Input: dimensioned drawing with shaded views. Units: mm. Origin: part minimum x, y, z. A direction names the side the tool comes from. Coordinates: 2 decimals unless noted, no trailing zeros. Loops run counter-clockwise (first coordinate to the right, second up) from the corner with the lowest first, then second, coordinate; pieces in that order, holes last.
Item 1: Line query: probe 1 along Z at (x, y) = (30.5, 32); probe 2 along Y at (x, z) = (18.5, 22); probe 3 along Z at (x, y) = (30, 19) (1 decimal). Output: solid intervals per line, ascending.
Item 2: Reachability of the marked faces 1, 2 and 3 from +Z, -Z, +X, -X, +Y, -Y: full face, straight path, thin tool, end or side. Return the list, or none.
Item 3: Section query A-A, the plane x = 33. Return the cut outline in (y, z) (1 decimal).
Item 4: Section query C-C, the plane z = 11. Return the cut outline in (x, y), then the cut area to 3 significant figures.
Item 5: Pin query (flat end, axial travel): pin 1 Ø3.5 at (x, y) = (3.54, 32.75) entering from +Z; pin 2 Ø6 at (x, z) = (7, 7.5) entering from +Y; pin 3 Ø1 at (y, z) = (5, 7.5) entering from -X (1 decimal); pin 4 Ø1.9 at (x, y) = (32.75, 3.54) entering from +Z. Return the tip coordinate at first contact, or that it passes through.
Item 6: Section query D-D, the plane z = 24. Return the cut outline in (x, y).
Item 7: Section query B-B, the plane z = 15.5. Return the cut outline in (x, y).
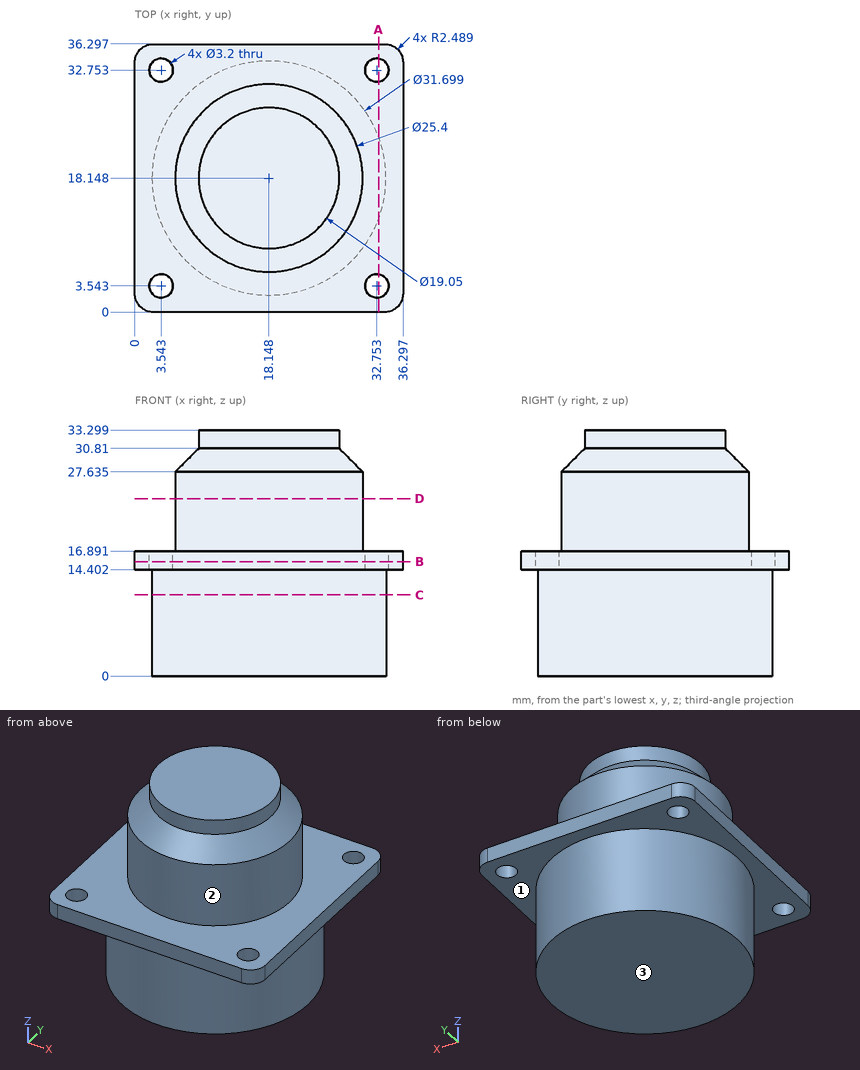
Verdict:
1. probe 1: z = 14.4 to 16.89
1. probe 2: y = 5.45 to 30.84
1. probe 3: z = 0 to 28.5
2. face 1: -Z
2. face 2: +Z
2. face 3: -Z, +X, -X, +Y, -Y
3. outline: (0, 14.4) - (2, 14.4) - (2, 16.9) - (0, 16.9) - close; (5.1, 14.4) - (12.6, 14.4) - (12.6, 0) - (23.7, 0) - (23.7, 14.4) - (31.2, 14.4) - (31.2, 16.9) - (5.1, 16.9) - close; (34.3, 14.4) - (36.3, 14.4) - (36.3, 16.9) - (34.3, 16.9) - close
4. outline: circle Ø31.7 at (18.15, 18.15)
4. area: 789 mm2
5. pin 1: stops at z = 16.89
5. pin 2: stops at y = 31.74
5. pin 3: stops at x = 8.6
5. pin 4: passes through
6. outline: circle Ø25.4 at (18.15, 18.15)
7. outline: (0, 2.49) arc R2.49 ccw to (2.49, 0) - (33.81, 0) arc R2.49 ccw to (36.3, 2.49) - (36.3, 33.81) arc R2.49 ccw to (33.81, 36.3) - (2.49, 36.3) arc R2.49 ccw to (0, 33.81) - close; hole circle Ø3.2 at (3.54, 3.54); hole circle Ø3.2 at (3.54, 32.75); hole circle Ø3.2 at (32.75, 3.54); hole circle Ø3.2 at (32.75, 32.75)
